Autodesk Fusion 360 part; units mm, degrees
sketch "Sketch1" plane through (0, 0, 0) normal (0, 0, 1) x (1, 0, 0)
  circle A0 centre (0, 0) radius 10
  line L0 (0, 0) -> (-50, 0) construction
  circle A1 centre (-50, 0) radius 10
  arc A2 (-39.7059, 14.1521) -> (-10.2941, 14.1521) centre (-25, 34.3693) ccw
  line L1 (9.4868, -28.4605) -> (9.4868, -40.9605)
  line L2 (-50, 0) -> (-50, 17.5) construction
  line L3 (-50, 17.5) -> (0, 17.5) construction
  line L4 (-25, 17.5) -> (-25, -94.314) construction
  line L5 (-25, -94.314) -> (-20, -94.314)
  line L6 (-25, -94.314) -> (-30, -94.314)
  line L7 (-20, -94.314) -> (-20, -52.314)
  line L8 (-30, -94.314) -> (-30, -52.314)
  line L9 (-20, -52.314) -> (-15, -52.314)
  line L10 (-30, -52.314) -> (-35, -52.314)
  arc A3 (-35, -52.314) -> (-53.163, -17.2118) centre (-57.6816, -41.8) ccw
  arc A4 (3.163, -17.2118) -> (-15, -52.314) centre (7.6816, -41.8) ccw
  arc A5 (-39.7059, 14.1521) -> (-53.163, -17.2118) centre (-50, 0) ccw
  arc A6 (3.163, -17.2118) -> (-10.2941, 14.1521) centre (0, 0) ccw
  dimension "d6" = 20
  dimension "d7" = 35
  dimension "d8" = 50
  dimension "d9" = 20
  dimension "d10" = 35
  dimension "d11" = 50
  dimension "d14" = 111.814
  dimension "d15" = 5
  dimension "d16" = 5
  dimension "d17" = 42
  dimension "d18" = 42
  dimension "d19" = 5
  dimension "d20" = 5
  dimension "d22" = 50
  dimension "d23" = 50
extrude "Extrude1" add sketch "Sketch1" along normal blind 20
Geometry: final body of the model. Coordinates: model frame, mm. A direction names the side the tool comes from. Give positions to 0.01 mm unless a question says otherwise; leave off trailing zeros. Write each loop counter-clockwise with the first axis right and the second up, starting at its lowest first coordinate (ties: lowest second). Pieces come first, ordered by that corner, then holes. Notation, with made-up numbers: (74.5, 33.25) -> (89.5, 33.25) arc R21 ccw to (89.5, 49.25) -> close; hole circle Ø4 at (-23, -9.75). An arc over 180 degrees is marked (long way). Answer in a Markdown table with one row per item.
(1) Section query C-C on x = -57. Return loops of the section in (y, z), then the cut area to 3 significant figures.
Answers below:
| item | result |
|---|---|
| outline | (-16.04, 0) -> (-7.14, 0) -> (-7.14, 20) -> (-16.04, 20) -> close; (7.14, 0) -> (16.04, 0) -> (16.04, 20) -> (7.14, 20) -> close |
| area | 356 mm^2 |
(2) Section query A-A on z = 4.25. Return loops of the section in (x, y).
Answers below:
| item | result |
|---|---|
| outline | (-53.16, -17.21) arc R25 cw to (-35, -52.31) -> (-30, -52.31) -> (-30, -94.31) -> (-20, -94.31) -> (-20, -52.31) -> (-15, -52.31) arc R25 cw to (3.16, -17.21) arc R17.5 ccw (long way) to (-10.29, 14.15) arc R25 cw to (-39.71, 14.15) arc R17.5 ccw (long way) to start; hole circle Ø20 at (-50, 0); hole circle Ø20 at (0, 0) |
(3) Section query B-B on y = 0. Return loops of the section in (x, z).
Answers below:
| item | result |
|---|---|
| outline | (-67.5, 0) -> (-60, 0) -> (-60, 20) -> (-67.5, 20) -> close; (-40, 0) -> (-10, 0) -> (-10, 20) -> (-40, 20) -> close; (10, 0) -> (17.5, 0) -> (17.5, 20) -> (10, 20) -> close |
(4) Set-up query: faces 5 (the flat face through (-18, -52.314, 10)), 6 (the flat face through (-30, -74, 10)), 7 (the cylindrical face through (-14.67, -30.6, 9.86)). Return all of +Z, -Z, +X, -X, +Y, -Y with unobstructed straight access to the full face (end or side cutting, diameter ignored); none if empty.
Answers below:
| item | result |
|---|---|
| face 5 | +Z, -Z, +X, -Y |
| face 6 | +Z, -Z, -X, -Y |
| face 7 | +Z, -Z, +X |
(5) Section query D-D on y = -75. Return loops of the section in (x, z), then the cut area to 3 significant figures.
Answers below:
| item | result |
|---|---|
| outline | (-30, 0) -> (-20, 0) -> (-20, 20) -> (-30, 20) -> close |
| area | 200 mm^2 |
(6) Draft query along Y for faces 1 (the cylindrical face through (-2.17, 9.76, 9.86)), 2 (the cylindrical face through (-66.25, 6.49, 9.86)), 3 (the cylindrical face through (-35.626, -30.029, 9.86)), 4 (the flat face through (-28, -17, 0)). Return one class per face: +Y half, -Y half, draft (parallel to the pull), parting line (faces both ways), or undercut.
Answers below:
| item | result |
|---|---|
| face 1 | undercut |
| face 2 | parting line |
| face 3 | undercut |
| face 4 | draft |
(7) Ray query, line 1 along Y through (x, z) = (-9, 3.5); line 2 along X through (y, z) = (1, 19); line 3 along Y through (x, z) = (2, 16.5). Return the intervals inside material, ascending. Write a range as [from, to].
Answers below:
| item | result |
|---|---|
| line 1 | [-23.18, -4.36], [4.36, 15.01] |
| line 2 | [-67.47, -59.95], [-40.05, -9.95], [9.95, 17.47] |
| line 3 | [-17.45, -9.8], [9.8, 17.39] |
(8) Pin query (flat end, axial travel): pin 1 (2 mm diameter, centred on x = -7, z = 11, fed in from -Y); pin 2 (12 mm diameter, centred on x = -50, y = 0, fed in from +Z); pin 3 (1.5 mm diameter, centred on y = -31, z = 13.5, fed in from +X); pin 4 (1.5 mm diameter, centred on y = -28.5, z = 17.5, fed in from -X). Return the tip coordinate at first contact, or that it passes through.
Answers below:
| item | result |
|---|---|
| pin 1 | y = -22.33 |
| pin 2 | through |
| pin 3 | x = -14.49 |
| pin 4 | x = -37 |
